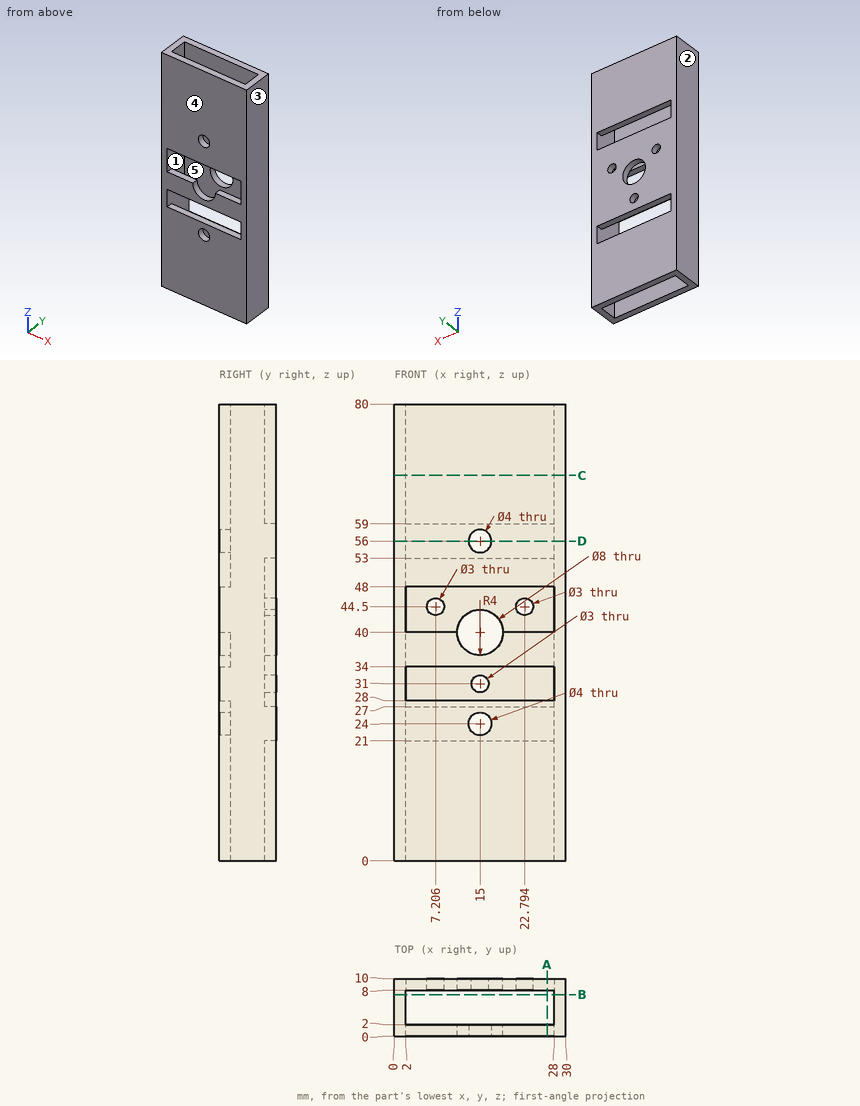
Here's the drawing with two shaded views (mm, measured from the low corner). I have some questions. A direction names the side the tool comes from. Coordinates: 2 decimals unless noted, no trailing zeros. Loops run counter-clockwise (first coordinate to the right, second up) from the corner with the lowest first, then second, coordinate; pieces in that order, holes last. Notation, with made-up numbers: (-23.5, 84) -> (33.5, 84) arc R31 cw to (33.5, 108) -> close; hole circle Ø3 at (32.5, 44.25). An arc over 180 degrees is marked (long way). Put each result on its own line as item: value. Start each with the question number.
Q1. I'm going to push flat-ended pins straight in: P1, Ø1, axis at x = 20, y = 1, coming from the -Z side; P2, Ø5, axis at x = 22.79, z = 44.5, coming from the -Y side. Where does each tip first touch, or does it pass through?
Q2. I want a section at B-B (y = 7.25). Write out the boundary of the cut face in (x, z).
Q3. I want a section at A-A (x = 26.75). Write out the boundary of the cut face in (y, z).
Q4. I want a section at C-C (z = 67.5). Write out the boundary of the cut face in (x, y), plus the area to 3 significant figures.
Q5. For the marked faces 1 and 2, which set-ups out of +Z, -Z, +X, -X, +Y, -Y let a thin tool reach every point of the face, with its end or its side?
Q6. If I drill on line 1 (X direction, y = 8.65, z = 44.5); line 2 (Z direction, x = 19.5, y = 0.75); line 3 (Z direction, x = 10.5, y = 9.75), over which ranges is the centre line in solid material (lowest first)? Write a range as [from, to].
Q7. I want a section at D-D (z = 56). Write out the boundary of the cut face in (x, y), plus the area to 3 significant figures.
Q8. Thinking about a two-plate mould opening in Y: for the marked faces 3, 4 and 5, which applies, pulls with the +Y half, pulls with the -Y half, needs draft (parallel to the pull), parting line crosses it, or undercut?
Taken from the geometry:
1. P1: stops at z = 0
1. P2: stops at y = 8
2. outline: (0, 0) -> (2, 0) -> (2, 80) -> (0, 80) -> close; (28, 0) -> (30, 0) -> (30, 80) -> (28, 80) -> close
3. outline: (0, 0) -> (2, 0) -> (2, 28) -> (0, 28) -> close; (0, 34) -> (2, 34) -> (2, 40) -> (0, 40) -> close; (0, 48) -> (2, 48) -> (2, 80) -> (0, 80) -> close; (8, 0) -> (10, 0) -> (10, 21) -> (8, 21) -> close; (8, 27) -> (10, 27) -> (10, 53) -> (8, 53) -> close; (8, 59) -> (10, 59) -> (10, 80) -> (8, 80) -> close
4. outline: (0, 0) -> (30, 0) -> (30, 10) -> (0, 10) -> close; hole (2, 2) -> (28, 2) -> (28, 8) -> (2, 8) -> close
4. area: 144 mm2
5. face 1: none
5. face 2: +Z, -Z, -X, +Y, -Y
6. line 1: x = [0, 5.71], [8.71, 21.29], [24.29, 30]
6. line 2: z = [0, 28], [34, 40], [48, 80]
6. line 3: z = [0, 21], [27, 53], [59, 80]
7. outline: (0, 0) -> (13, 0) -> (13, 2) -> (2, 2) -> (2, 10) -> (0, 10) -> close; (17, 0) -> (30, 0) -> (30, 10) -> (28, 10) -> (28, 2) -> (17, 2) -> close
7. area: 84.0 mm2
8. face 3: needs draft
8. face 4: pulls with the -Y half
8. face 5: undercut
